Geometry check sheet. Reference: the model listing, model coordinates, mm. Face numbers are marked on the shaded views. Give positions to 0.01 mm unless a question says otherwise; leave off trailing zeros. Loops run counter-clockwise (first coordinate to the right, second up) from the corner with the lowest first, then second, coordinate; pieces in that order, holes last. Notation, with made-up numbers: (-19.75, 78.25) - (-11.75, 78.25) arc R22 cw to (-11.75, 117.25) - close; hole circle Ø8 at (-29.5, -12.5). An arc over 180 degrees is marked (long way). One line per question, with ' | ' between items. Start each with the question number.
from build123d import *
from OCP.BRepFilletAPI import BRepFilletAPI_MakeChamfer

# Parameters (mm, degrees)
SKETCH1_W           = 28
SKETCH1_H           = 16
BOSS_EXTRUDE1_DEPTH = 2
CHAMFER1_SIZE       = 1
CHAMFER1_SIZE2      = 1.035530314
SKETCH1_3_W         = 2
SKETCH1_3_H         = 7.9
BOSS_EXTRUDE2_DEPTH = 7
CUT_EXTRUDE1_DEPTH  = 20.692701694
SKETCH2_3_R         = 0.5
BOSS_EXTRUDE3_DEPTH = 7.9
FILLET1_R           = 2


with BuildPart() as part:
    # Sketch1 → Boss-Extrude1 (new body)
    with BuildSketch(Plane(origin=(0, 0, 0), x_dir=(1, 0, 0), z_dir=(0, 1, 0))):
        Rectangle(SKETCH1_W, SKETCH1_H)
    extrude(amount=BOSS_EXTRUDE1_DEPTH)

    # Chamfer1: one chamfer whose edges measure the first distance from different faces: ONE call of the kernel's chamfer builder (chamfer() names one face for all edges)
    chamfer1_edges_1 = [part.edges().sort_by_distance(p)[0] for p in [
        (14, 2, 0),
    ]]
    chamfer1_side_1 = [part.faces().sort_by_distance(p)[0] for p in [
        (0, 2, 0),
    ]]
    chamfer1_edges_2 = [part.edges().sort_by_distance(p)[0] for p in [
        (-14, 2, 0),
    ]]
    chamfer1_side_2 = [part.faces().sort_by_distance(p)[0] for p in [
        (-14, 1, 0),
    ]]
    chamfer1 = BRepFilletAPI_MakeChamfer(part.part.solid().wrapped)
    for e in chamfer1_edges_1:
        chamfer1.Add(CHAMFER1_SIZE, CHAMFER1_SIZE2, e.wrapped, chamfer1_side_1[0].wrapped)  # the first distance lies on this face
    for e in chamfer1_edges_2:
        chamfer1.Add(CHAMFER1_SIZE, CHAMFER1_SIZE2, e.wrapped, chamfer1_side_2[0].wrapped)  # the first distance lies on this face
    add(Compound.cast(chamfer1.Shape()), mode=Mode.REPLACE)

    # Sketch1<3> → Boss-Extrude2 (add)
    with BuildSketch(Plane(origin=(0, 0, 0), x_dir=(1, 0, 0), z_dir=(0, 1, 0))):
        with Locations((-5.95, 0)):
            Rectangle(SKETCH1_3_W, SKETCH1_3_H)
        with Locations((5.95, 0)):
            Rectangle(SKETCH1_3_W, SKETCH1_3_H)
    extrude(amount=BOSS_EXTRUDE2_DEPTH)

    # Sketch2 → Cut-Extrude1 (cut, through all)
    with BuildSketch(Plane.XY.offset(3.95)):
        Polygon((-6.95, 7), (-6.95, 5.430500874), (-5.95, 7), align=None)
        with BuildLine():
            Line((7.45, 4.5), (7.45, 7))
            Line((7.45, 7), (5.95, 7))
            Line((5.95, 7), (7.371681261, 4.768672504))
            ThreePointArc((7.371681261, 4.768672504), (7.430021161, 4.639927427), (7.45, 4.5))
        make_face()
    extrude(amount=-CUT_EXTRUDE1_DEPTH, mode=Mode.SUBTRACT)

    # Sketch2<3> → Boss-Extrude3 (add)
    with BuildSketch(Plane.XY.offset(3.95)):
        with BuildLine():
            ThreePointArc((-6.95, 5), (-7.190482586, 4.938369851), (-7.371681261, 4.768672504))
            ThreePointArc((-7.371681261, 4.768672504), (-7.430021161, 4.639927427), (-7.45, 4.5))
            ThreePointArc((-7.45, 4.5), (-7.303553391, 4.146446609), (-6.95, 4))
            Line((-6.95, 4), (-6.95, 5))
        make_face()
        with BuildLine():
            ThreePointArc((-6.45, 4.5), (-6.596446609, 4.853553391), (-6.95, 5))
            Line((-6.95, 5), (-6.95, 4))
            ThreePointArc((-6.95, 4), (-6.596446609, 4.146446609), (-6.45, 4.5))
        make_face()
        with BuildLine():
            Line((-6.95, 5.430500874), (-7.371681261, 4.768672504))
            ThreePointArc((-7.371681261, 4.768672504), (-7.190482586, 4.938369851), (-6.95, 5))
            Line((-6.95, 5), (-6.95, 5.430500874))
        make_face()
        with Locations((6.95, 4.5)):
            Circle(SKETCH2_3_R)
        with BuildLine():
            Line((7.371681261, 4.768672504), (5.95, 7))
            Line((5.95, 7), (5.95, 4.5))
            Line((5.95, 4.5), (6.45, 4.5))
            ThreePointArc((6.45, 4.5), (6.810072573, 4.980021161), (7.371681261, 4.768672504))
        make_face()
    extrude(amount=-BOSS_EXTRUDE3_DEPTH)

    # Fillet1
    fillet1_edges = [part.edges().sort_by_distance(p)[0] for p in [
        (5.45, 7, -3.95),
        (5.45, 7, 3.95),
        (-5.45, 7, 3.95),
        (-5.45, 7, -3.95),
    ]]
    fillet(fillet1_edges, radius=FILLET1_R)


solid = part.part
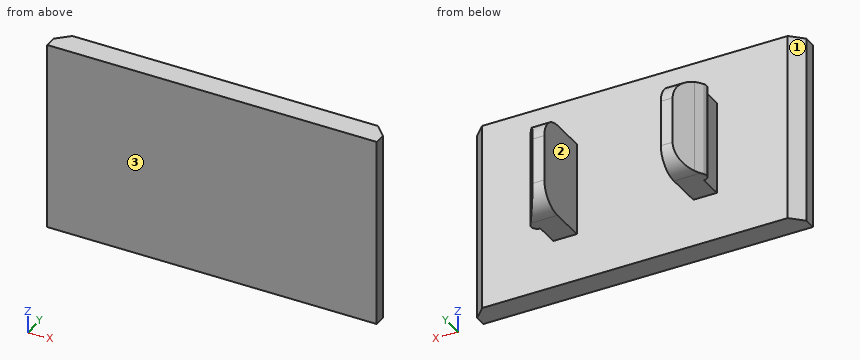
(1) Section check D-D, the plane y = 5.75. Record the boundary of the cut face in (x, z), and give its area (3 significant figures).
(2) Depth check by flat-ended pin: pin 1 Ø2 at (y, z) = (2.5, 4.5) entering from -X; pin 2 Ø1.5 at (x, z) = (7, -1) entering from +Y; pin 3 Ø4 at (x, y) = (8.5, 5.5) entering from -Z. Enter the tip coordinate at first touch or a pass-through.
(3) Mould release check, pull along X, two halves, no side actions. Record for the marked faces 1, 2 and 3: pulls with the +X half, pulls with the -X half, needs draft (parallel to the pull), parting line crosses it, or undercut.
(4) Material ranges on line 1 (X direction, y = 3.25, z = -3.5); line 2 (Y direction, x = 0.25, z = -7.5); line 3 (Y direction, x = -7.25, z = -3.25), recorded low to high.
(5) Section check A-A, the plane y = 3. Record the boundary of the cut face in (x, z).
(6) Section check C-C, the plane x = 9. Record the boundary of the cut face in (y, z).
(7) Section check B-B, the plane z = 1.5. Record the boundary of the cut face in (x, y).
Numbers:
1) outline: (-6.75, -3.8) - (-4.95, -3.8) - (-4.95, 3.8) - (-6.75, 3.8) - close; (4.95, -3.8) - (6.75, -3.8) - (6.75, 3.8) - (4.95, 3.8) - close | area: 27.3 mm^2
2) pin 1: x = -13.48 | pin 2: y = 6.53 | pin 3: z = -3.95
3) face 1: pulls with the -X half | face 2: undercut | face 3: needs draft
4) line 1: -6.95 to -4.95, 4.95 to 6.95 | line 2: 0 to 2 | line 3: 0 to 2, 4.1 to 4.96
5) outline: (-6.95, -3.95) - (-4.95, -3.95) - (-4.95, 3.95) - (-6.95, 3.95) - close; (4.95, -3.95) - (6.95, -3.95) - (6.95, 3.95) - (4.95, 3.95) - close
6) outline: (0, -8) - (2, -8) - (2, 8) - (0, 8) - close
7) outline: (-14, 0) - (14, 0) - (14, 0.96) - (13, 2) - (6.95, 2) - (6.95, 4) arc R0.5 ccw to (7.37, 4.77) - (5.95, 7) - (4.95, 7) - (4.95, 2) - (-4.95, 2) - (-4.95, 7) - (-5.95, 7) - (-7.37, 4.77) arc R0.5 ccw to (-6.95, 4) - (-6.95, 2) - (-12.96, 2) - (-14, 1) - close
